Work out the finished part from the listing and answer in its coordinate system (mm). Face numbers are marked on the shaded views. A direction names the side the tool comes from. Coordinates: 2 decimals unless noted, no trailing zeros. Loops run counter-clockwise (first coordinate to the right, second up) from the corner with the lowest first, then second, coordinate; pieces in that order, holes last. Notation, with made-up numbers: (-20, -27) - (0, -27) arc R12 cw to (0, -22) - close; hole circle Ø5 at (40, -3). An arc over 180 degrees is marked (long way). Write each question's results on one line, items separated by ' | '. Start each with the question number.
1. A cutting plane is placed at C-C on y = 12.5. Determine the outline of the cut face in (x, z), then the cut area to 3 significant figures.
2. A cutting plane is placed at A-A on z = 0. Determine the outline of the cut face in (x, y), then the cut area to 3 significant figures.
3. Determine the mould class of the marked faces 4, 5 and 6 for opening direction Z: released by +Z, released by -Z, zero draft, split by the parting line, or undercut.
4. Each of these flat-tipped pins is pushed along its axis until it touches: P1, Ø1.5, axis at x = -84.5, y = 10.5, coming from the -Z side; P2, Ø4.5, axis at y = 15.5, z = -1.5, coming from the -X side; P3, Ø12, axis at x = -31, y = 21, coming from the -Z side. Where does it stop, or does it pass through?
5. A cutting plane is placed at B-B on x = 0. Determine the outline of the cut face in (y, z).
6. Which of the six approach directions +Z, -Z, +X, -X, +Y, -Y give full straight-line access (tool end or side, diameter ignored) to the marked faces 1, 2 and 3?
7. Find the intervals of material crossed by line 1 along Y through (x, z) = (-88, 0); line 2 along Z through (x, y) = (1, 4.25); line 3 along X through (y, z) = (10, -2.5), in increasing order. Write a range as [from, to].
8. A cutting plane is placed at D-D on z = -15.5. Determine the outline of the cut face in (x, y).
from build123d import *

# Parameters (mm, degrees)
SKETCH1_W           = 45
SKETCH1_H           = 39
SKETCH1_W_2         = 25
SKETCH1_H_2         = 19
EXTRUDE_THIN1_DEPTH = 25
FILLET1_R           = 10
FILLET2_R           = 4
SKETCH2_R           = 11
BOSS_EXTRUDE1_DEPTH = 75
SKETCH3_R           = 7.85
CUT_EXTRUDE1_DEPTH  = 30


with BuildPart() as part:
    # Sketch1 → Extrude-Thin1 (new body)
    with BuildSketch(Plane(origin=(0, 0, 0), x_dir=(1, 0, 0), z_dir=(0, 1, 0))):
        Rectangle(SKETCH1_W, SKETCH1_H)
        Rectangle(SKETCH1_W_2, SKETCH1_H_2, mode=Mode.SUBTRACT)
    extrude(amount=EXTRUDE_THIN1_DEPTH)

    # Fillet1
    fillet1_edges = [part.edges().sort_by_distance(p)[0] for p in [
        (22.5, 12.5, 19.5),
        (-22.5, 12.5, 19.5),
        (-22.5, 12.5, -19.5),
        (22.5, 12.5, -19.5),
    ]]
    fillet(fillet1_edges, radius=FILLET1_R)

    # Fillet2
    fillet2_edges = [part.edges().sort_by_distance(p)[0] for p in [
        (12.5, 12.5, 9.5),
        (12.5, 12.5, -9.5),
        (-12.5, 12.5, -9.5),
        (-12.5, 12.5, 9.5),
    ]]
    fillet(fillet2_edges, radius=FILLET2_R)

    # Sketch2 → Boss-Extrude1 (add)
    with BuildSketch(Plane(origin=(-22.5, 0, 3), x_dir=(0, 0, 1), z_dir=(-1, 0, 0))):
        with Locations((-3, 12.5)):
            Circle(SKETCH2_R)
    extrude(amount=BOSS_EXTRUDE1_DEPTH)

    # Sketch3 → Cut-Extrude1 (cut)
    with BuildSketch(Plane.ZY.offset(97.5)):
        with Locations((0, 12.5)):
            Circle(SKETCH3_R)
    extrude(amount=-CUT_EXTRUDE1_DEPTH, mode=Mode.SUBTRACT)


solid = part.part
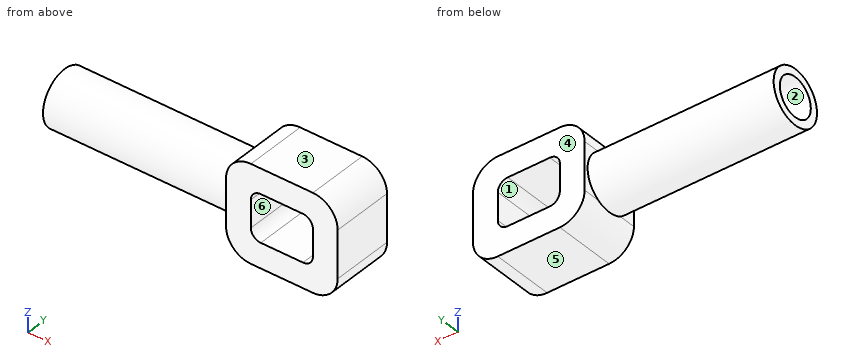
Values:
1) outline: (-97.5, -11) - (-22.5, -11) - (-22.5, -9.5) arc R10 ccw to (-12.5, -19.5) - (12.5, -19.5) arc R10 ccw to (22.5, -9.5) - (22.5, 9.5) arc R10 ccw to (12.5, 19.5) - (-12.5, 19.5) arc R10 ccw to (-22.5, 9.5) - (-22.5, 11) - (-97.5, 11) - (-97.5, 7.85) - (-67.5, 7.85) - (-67.5, -7.85) - (-97.5, -7.85) - close; hole (-12.5, -5.5) arc R4 ccw to (-8.5, -9.5) - (8.5, -9.5) arc R4 ccw to (12.5, -5.5) - (12.5, 5.5) arc R4 ccw to (8.5, 9.5) - (-8.5, 9.5) arc R4 ccw to (-12.5, 5.5) - close | area: 2,390 mm^2
2) outline: (-97.5, 1.5) - (-22.5, 1.5) - (-22.5, 0) - (-12.5, 0) - (-12.5, 25) - (-22.5, 25) - (-22.5, 23.5) - (-97.5, 23.5) - (-97.5, 20.35) - (-67.5, 20.35) - (-67.5, 4.65) - (-97.5, 4.65) - close; (12.5, 0) - (22.5, 0) - (22.5, 25) - (12.5, 25) - close | area: 1,680 mm^2
3) face 4: zero draft | face 5: released by -Z | face 6: undercut
4) P1: z = -10.93 | P2: x = -67.5 | P3: z = -10.71
5) outline: (0, -19.5) - (25, -19.5) - (25, -9.5) - (0, -9.5) - close; (0, 9.5) - (25, 9.5) - (25, 19.5) - (0, 19.5) - close
6) face 1: +Y, -Y | face 2: -X | face 3: +Z, +X, -X, +Y, -Y
7) line 1: [1.5, 4.65], [20.35, 23.5] | line 2: [-19.5, -9.5], [9.5, 19.5] | line 3: [-67.5, -12.5], [12.5, 22.5]
8) outline: (-20.5, 0) - (20.5, 0) - (20.5, 25) - (-20.5, 25) - close
